Geometry check sheet. Reference: the model listing, model coordinates, mm. Face numbers are marked on the shaded views. A direction names the side the tool comes from. Give positions to 0.01 mm unless a question says otherwise; leave off trailing zeros. Write each loop counter-clockwise with the first axis right and the second up, starting at its lowest first coordinate (ties: lowest second). Pieces come first, ordered by that corner, then holes. Notation, with made-up numbers: (-27, -36) -> (6, -36) arc R22 cw to (6, -25) -> close; hole circle Ø10 at (12, 11.5). An arc over 180 degrees is marked (long way). Use a Markdown table: item, result. Add a question column.
from build123d import *

# Parameters (mm, degrees)
SKIZZE1_R                                            = 1.385
AUFSATZ_LINEAR_AUSTRAGEN1_DEPTH                      = 6.74
AUFSATZ_LINEAR_AUSTRAGEN1_DEPTH_BACK                 = 3.42
SKIZZE2_W                                            = 16.035180953
SKIZZE2_H                                            = 1.68
SCHNITT_LINEAR_AUSTRAGEN1_DEPTH                      = 14.21
SCHNITT_LINEAR_AUSTRAGEN1_DEPTH_BACK                 = 14.21
SKIZZE3_R                                            = 1.2
SCHNITT_LINEAR_AUSTRAGEN2_DEPTH                      = 2.16
SKIZZE4_R                                            = 0.35
AUFSATZ_LINEAR_AUSTRAGEN2_DEPTH                      = 4
LINEAR_AUSTRAGEN_D_NN1_DEPTH                         = 0.55
FORMSENKUNG_F_R_M3_SENKSCHRAUBE_MIT_SCHL_D           = 3
FORMSENKUNG_F_R_M3_SENKSCHRAUBE_MIT_SCHL_DEPTH       = 11
FORMSENKUNG_F_R_M3_SENKSCHRAUBE_MIT_SCHL_CSINK_D     = 5.6
FORMSENKUNG_F_R_M3_SENKSCHRAUBE_MIT_SCHL_CSINK_ANGLE = 90
FORMSENKUNG_F_R_M3_SENKSCHRAUBE_MIT_SCHL_TIP         = 0.901290929


with BuildPart() as part:
    # Skizze1 → Aufsatz-Linear austragen1 (new body, two sides)
    with BuildSketch(Plane(origin=(0, 0, 0), x_dir=(1, 0, 0), z_dir=(0, 1, 0))) as aufsatz_linear_austragen1_sk:
        Polygon((-13.21, -18.65), (-13.21, -12.79), (-7.6, -7.09), (7.6, -7.09), (13.21, -12.79), (13.21, -18.65), align=None)
        with Locations((-10.48, -15.75)):
            Circle(SKIZZE1_R, mode=Mode.SUBTRACT)
        with Locations((10.48, -15.75)):
            Circle(SKIZZE1_R, mode=Mode.SUBTRACT)
    extrude(amount=AUFSATZ_LINEAR_AUSTRAGEN1_DEPTH)
    extrude(aufsatz_linear_austragen1_sk.sketch, amount=-AUFSATZ_LINEAR_AUSTRAGEN1_DEPTH_BACK)

    # Skizze2 → Schnitt-Linear austragen1 (cut, two sides)
    with BuildSketch(Plane(origin=(0, 0, 0), x_dir=(0, 0, -1), z_dir=(1, 0, 0))) as schnitt_linear_austragen1_sk:
        with Locations((-5.332409524, 0.44)):
            Rectangle(SKIZZE2_W, SKIZZE2_H)
    extrude(amount=SCHNITT_LINEAR_AUSTRAGEN1_DEPTH, mode=Mode.SUBTRACT)
    extrude(schnitt_linear_austragen1_sk.sketch, amount=-SCHNITT_LINEAR_AUSTRAGEN1_DEPTH_BACK, mode=Mode.SUBTRACT)

    # Skizze3 → Schnitt-Linear austragen2 (cut)
    with BuildSketch(Plane(origin=(0, 6.74, 0), x_dir=(1, 0, 0), z_dir=(0, 1, 0))):
        with Locations((6.35, -15.75)):
            Circle(SKIZZE3_R)
        with Locations((-6.35, -15.75)):
            Circle(SKIZZE3_R)
    extrude(amount=-SCHNITT_LINEAR_AUSTRAGEN2_DEPTH, mode=Mode.SUBTRACT)

    # Skizze4 → Aufsatz-Linear austragen2 (add)
    with BuildSketch(Plane.XY.offset(18.65)):
        with Locations((0, -1.9)):
            Circle(SKIZZE4_R)
        with Locations((2.54, -1.9)):
            Circle(SKIZZE4_R)
        with Locations((5.08, -1.9)):
            Circle(SKIZZE4_R)
        with Locations((-2.54, -1.9)):
            Circle(SKIZZE4_R)
        with Locations((-5.08, -1.9)):
            Circle(SKIZZE4_R)
    extrude(amount=AUFSATZ_LINEAR_AUSTRAGEN2_DEPTH)

    # Skizze5 → Linear-Austragen-Dünn1 (add, symmetric)
    with BuildSketch(Plane(origin=(8.1, 0, 0), x_dir=(0, 0, -1), z_dir=(1, 0, 0))):
        with BuildLine():
            Line((-18.65, -1.57), (-20.15, -1.57))
            ThreePointArc((-20.15, -1.57), (-20.609619408, -1.379619408), (-20.8, -0.92))
            Line((-20.8, -0.92), (-20.8, 3.58))
            ThreePointArc((-20.8, 3.58), (-20.609619408, 4.039619408), (-20.15, 4.23))
            Line((-20.15, 4.23), (-18.65, 4.23))
            Line((-18.65, 4.23), (-18.65, 4.93))
            Line((-18.65, 4.93), (-20.15, 4.93))
            ThreePointArc((-20.15, 4.93), (-21.104594155, 4.534594155), (-21.5, 3.58))
            Line((-21.5, 3.58), (-21.5, -0.92))
            ThreePointArc((-21.5, -0.92), (-21.104594155, -1.874594155), (-20.15, -2.27))
            Line((-20.15, -2.27), (-18.65, -2.27))
            Line((-18.65, -2.27), (-18.65, -1.57))
        make_face()
    linear_austragen_d_nn1 = extrude(amount=LINEAR_AUSTRAGEN_D_NN1_DEPTH, both=True)

    # Spiegeln1: Linear-Austragen-Dünn1 across plane
    add(linear_austragen_d_nn1.mirror(Plane(origin=(0, 0, 0), x_dir=(0, 0, 1), z_dir=(1, 0, 0))))

    # Formsenkung für M3 Senkschraube mit Schlitz/Kreuzschlitz1
    with Locations(Plane(origin=(0, -3.42, 0), x_dir=(-1, 0, 0), z_dir=(0, -1, 0))):
        with Locations((-10.48, -15.75), (10.48, -15.75)):
            CounterSinkHole(FORMSENKUNG_F_R_M3_SENKSCHRAUBE_MIT_SCHL_D / 2, FORMSENKUNG_F_R_M3_SENKSCHRAUBE_MIT_SCHL_CSINK_D / 2, depth=FORMSENKUNG_F_R_M3_SENKSCHRAUBE_MIT_SCHL_DEPTH, counter_sink_angle=FORMSENKUNG_F_R_M3_SENKSCHRAUBE_MIT_SCHL_CSINK_ANGLE)
            with Locations((0, 0, -(FORMSENKUNG_F_R_M3_SENKSCHRAUBE_MIT_SCHL_DEPTH + FORMSENKUNG_F_R_M3_SENKSCHRAUBE_MIT_SCHL_TIP / 2))):  # 118° drill point
                Cone(0, FORMSENKUNG_F_R_M3_SENKSCHRAUBE_MIT_SCHL_D / 2, FORMSENKUNG_F_R_M3_SENKSCHRAUBE_MIT_SCHL_TIP, mode=Mode.SUBTRACT)


solid = part.part
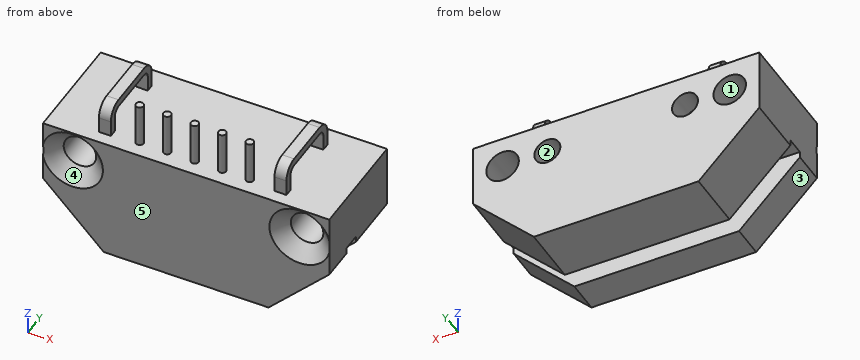
1) Tool access check on the marked faces 1 and 2. Record the directions out of +Z, -Z, +X, -X, +Y, -Y that give a thin tool (end or side, any length) a straight path to the whole face; none if there is none.
2) Material ranges on probe 1 along X at (y, z) = (6.15, 15.75); probe 2 along X at (y, z) = (3.75, 15.75); probe 3 along Z at (x, y) = (-10.48, 1), recorded low to high. Write a range as [from, to].
3) Draft check along Z on the marked faces 3, 4 and 5. Enter one of: +Z half, -Z half, draft (parallel to the pull), parting line (faces both ways), or undercut.
4) Sectioned sample at B-B, the plane z = 19. Count the separate pieces of the cut face and the enclosed holes in it, and give its area (3 significant figures).
5) Gauge pin test, flat ends, axial feed: P1, Ø4, axis at x = -10.48, z = 15.75, coming from the -Y side; P2, Ø2, axis at x = 9.5, z = 19.5, coming from the +Y side; P3, Ø1.2, axis at x = 8, z = 19.5, coming from the -Y side; P4, Ø0.9, axis at x = 8, y = 1.5, coming from the +Z side. Record the tip position at first contact, or that the pin passes through.
6) Sectioned sample at A-A, the plane y = 0.5. Enter the section's corners in (x, z), and give its area (3 significant figures).
7) Sectioned sample at C-C, the plane x = 10.48. Enter the section's corners in (y, z).
8) Sectioned sample at D-D, the plane x = -6.35. Enter the section's corners in (y, z), and give its area (3 significant figures).
Check values:
| question | item | result |
|---|---|---|
| 1 | face 1 | +Y, -Y |
| 1 | face 2 | +Y |
| 2 | probe 1 | [-13.21, -11.98], [-8.98, -7.55], [-5.15, 5.15], [7.55, 8.98], [11.98, 13.21] |
| 2 | probe 2 | [-13.21, -11.98], [-8.98, 8.98], [11.98, 13.21] |
| 2 | probe 3 | [13.35, 14.25], [17.25, 18.65] |
| 3 | face 3 | -Z half |
| 3 | face 4 | undercut |
| 3 | face 5 | draft |
| 4 | separate pieces | 9 |
| 4 | enclosed holes | 0 |
| 4 | area | 5.00 mm² |
| 5 | P1 | y = -2.62 |
| 5 | P2 | y = 6.74 |
| 5 | P3 | y = -2.27 |
| 5 | P4 | z = 21.5 |
| 6 | outline | (-13.21, 13.35) -> (13.21, 13.35) -> (13.21, 18.65) -> (-13.21, 18.65) -> close; (-8.65, 20.8) -> (-7.55, 20.8) -> (-7.55, 21.5) -> (-8.65, 21.5) -> close; (7.55, 20.8) -> (8.65, 20.8) -> (8.65, 21.5) -> (7.55, 21.5) -> close; hole circle Ø3 at (-10.48, 15.75); hole circle Ø3 at (10.48, 15.75) |
| 6 | area | 127 mm² |
| 7 | outline | (-3.42, 10.02) -> (-0.4, 10.02) -> (-0.4, 13.35) -> (1.28, 13.35) -> (1.28, 10.02) -> (6.74, 10.02) -> (6.74, 14.25) -> (-2.12, 14.25) -> (-3.42, 12.95) -> close; (-3.42, 18.55) -> (-2.12, 17.25) -> (6.74, 17.25) -> (6.74, 18.65) -> (-3.42, 18.65) -> close |
| 8 | outline | (-3.42, 7.09) -> (-0.4, 7.09) -> (-0.4, 13.35) -> (1.28, 13.35) -> (1.28, 7.09) -> (6.74, 7.09) -> (6.74, 14.55) -> (4.58, 14.55) -> (4.58, 16.95) -> (6.74, 16.95) -> (6.74, 18.65) -> (-3.42, 18.65) -> close |
| 8 | area | 102 mm² |
